```python
from build123d import *

# Parameters (mm, degrees)
MODEL_R                  = 1.6
MODEL_R_2                = 1.8
MODEL_R_3                = 4
MODEL_R_4                = 11.5
MODEL_W                  = 6.599987016
MODEL_H                  = 9.199995837
MODEL_W_2                = 6.600001917
MODEL_H_2                = 9.1999977
RESSALTO_EXTRUS_O1_DEPTH = 6


with BuildPart() as part:
    # Model → Ressalto-extrusão1 (new body)
    with BuildSketch(Plane.XY):
        Polygon((68.160504095, 58.4189533), (68.160504095, 53.118954478), (69.960502327, 53.118954478), (69.960502327, 48.018956714), (68.160504095, 48.018956714), (68.160504095, 44.068956891), (63.760499423, 44.068956891), (63.760499423, 48.018956714), (61.960501191, 48.018956714), (61.960501191, 53.118954478), (63.760499423, 53.118954478), (63.760499423, 58.4189533), (58.460502168, 58.4189533), (58.460502168, 62.768951191), (58.392353821, 63.286589281), (58.192552976, 63.768951191), (57.874715731, 64.183164754), (57.460502168, 64.501001999), (56.978140258, 64.700802844), (56.460502168, 64.768951191), (51.660507726, 64.768951191), (51.142869636, 64.700802844), (50.660507726, 64.501001999), (50.246294164, 64.183164754), (49.928456918, 63.768951191), (49.728656073, 63.286589281), (49.660507726, 62.768951191), (49.660507726, 58.4189533), (34.035520335, 58.4189533), (34.035520335, 13.418967617), (39.035518735, 8.418969217), (98.035493414, 8.418969027), (98.035488298, 58.4189533), (82.260492067, 58.4189533), (82.260492067, 62.768951191), (82.192343719, 63.286589281), (81.992542874, 63.768951191), (81.674705629, 64.183164754), (81.260492067, 64.501001999), (80.778130157, 64.700802844), (80.260492067, 64.768951191), (75.460496102, 64.768951191), (74.942858011, 64.700802844), (74.460496102, 64.501001999), (74.046282539, 64.183164754), (73.728445294, 63.768951191), (73.528644449, 63.286589281), (73.460496102, 62.768951191), (73.460496102, 58.4189533), align=None)
        with Locations((50.235508479, 44.618957639)):
            Circle(MODEL_R, mode=Mode.SUBTRACT)
        with Locations((50.235508479, 13.618967559)):
            Circle(MODEL_R, mode=Mode.SUBTRACT)
        with Locations((81.235498559, 13.618967559)):
            Circle(MODEL_R, mode=Mode.SUBTRACT)
        with Locations((81.235498559, 44.618957639)):
            Circle(MODEL_R, mode=Mode.SUBTRACT)
        with Locations((92.255495512, 33.418961223)):
            Circle(MODEL_R_2, mode=Mode.SUBTRACT)
        with Locations((39.215511525, 33.418961223)):
            Circle(MODEL_R_2, mode=Mode.SUBTRACT)
        with Locations((48.735508959, 29.118962599)):
            Circle(MODEL_R_3, mode=Mode.SUBTRACT)
        with Locations((65.735503519, 29.118962599)):
            Circle(MODEL_R_4, mode=Mode.SUBTRACT)
        with Locations((92.255493633, 45.318957274)):
            Rectangle(MODEL_W, MODEL_H, mode=Mode.SUBTRACT)
        with Locations((39.215512485, 45.318957274)):
            Rectangle(MODEL_W_2, MODEL_H, mode=Mode.SUBTRACT)
        with Locations((39.215512485, 21.518966444)):
            Rectangle(MODEL_W_2, MODEL_H_2, mode=Mode.SUBTRACT)
        with Locations((92.255493633, 21.518966444)):
            Rectangle(MODEL_W, MODEL_H_2, mode=Mode.SUBTRACT)
    extrude(amount=RESSALTO_EXTRUS_O1_DEPTH)


solid = part.part
```
Build history of the part. All positions in model axes, mm. A direction names the side the tool comes from. Coordinates: 2 decimals unless noted, no trailing zeros. Order: outer loops, then holes, each group sorted by start corner. A loop starts at its lowest first (then second) coordinate and runs counter-clockwise, first axis right, second up.
Item 1: Tool access for faces 4 (the flat face through (66, 44.069, 3)), 5 (the flat face through (54, 64.769, 3)), 6 (the flat face through (39, 26.119, 3)): list every direction of +Z, -Z, +X, -X, +Y, -Y with a clear straight run to the whole face (end or side of a thin tool).
Filled in:
face 4: +Z, -Z, +Y
face 5: +Z, -Z, +X, -X, +Y
face 6: +Z, -Z
Item 2: Saw through at C-C on x = 63. List the corners of the cut face in (y, z).
Filled in:
outline: (8.42, 0) - (17.95, 0) - (17.95, 6) - (8.42, 6) - close; (40.29, 0) - (48.02, 0) - (48.02, 6) - (40.29, 6) - close; (53.12, 0) - (58.42, 0) - (58.42, 6) - (53.12, 6) - close
Item 3: Drill centre lines: L1, parallel to X at y = 49, z = 2.7; L2, parallel to Y at x = 66, z = 4.15; L3, parallel to X at y = 18.5, z = 5.25. Where is each one in solid material? Low to high.
Filled in:
L1: x = 34.04 to 35.92, 42.52 to 61.96, 69.96 to 88.96, 95.56 to 98.04
L2: y = 8.42 to 17.62, 40.62 to 44.07
L3: x = 34.04 to 35.92, 42.52 to 61.32, 70.15 to 88.96, 95.56 to 98.04
Item 4: Drop flat-ended pins along their axis: pin 1 Ø2 at (x, z) = (66, 3.5) entering from +Y; pin 2 Ø0.9 at (x, z) = (63, 3) entering from +Y; pin 3 Ø2 at (y, z) = (61.5, 3.5) entering from -X. Give the stop position or say it passes through.
Filled in:
pin 1: stops at y = 44.07
pin 2: stops at y = 58.42
pin 3: stops at x = 49.66
Item 5: Saw through at B-B on x = 93. List the corners of the cut face in (y, z).
Filled in:
outline: (8.42, 0) - (16.92, 0) - (16.92, 6) - (8.42, 6) - close; (26.12, 0) - (31.78, 0) - (31.78, 6) - (26.12, 6) - close; (35.06, 0) - (40.72, 0) - (40.72, 6) - (35.06, 6) - close; (49.92, 0) - (58.42, 0) - (58.42, 6) - (49.92, 6) - close
Item 6: Saw through at D-D on y = 27. List the corners of the cut face in (x, z).
Filled in:
outline: (34.04, 0) - (45.34, 0) - (45.34, 6) - (34.04, 6) - close; (52.13, 0) - (54.43, 0) - (54.43, 6) - (52.13, 6) - close; (77.04, 0) - (98.04, 0) - (98.04, 6) - (77.04, 6) - close
Item 7: Saw through at A-A on y = 20.5. List the corners of the cut face in (x, z), then the cut area to 3 significant figures.
Filled in:
outline: (34.04, 0) - (35.92, 0) - (35.92, 6) - (34.04, 6) - close; (42.52, 0) - (58.12, 0) - (58.12, 6) - (42.52, 6) - close; (73.35, 0) - (88.96, 0) - (88.96, 6) - (73.35, 6) - close; (95.56, 0) - (98.04, 0) - (98.04, 6) - (95.56, 6) - close
area: 213 mm2
Item 8: Mould opens along Y. For faces 1 (the flat face through (98.035, 33, 3)), 2 (the cylindrical face through (40.932, 33.96, 2.958)), 3 (the flat face through (68, 8.419, 3)) say: released by +Y, released by -Y, zero draft, split by the parting line, or undercut.
Filled in:
face 1: zero draft
face 2: undercut
face 3: released by -Y
